Model file for the job. Use its own axes, mm. Round coordinates to 2 decimals unless told otherwise and drop trailing zeros. Loops run counter-clockwise (first coordinate to the right, second up) from the corner with the lowest first, then second, coordinate; pieces in that order, holes last. Notation, with made-up numbers: M 67.25,-37 L 87.25,-37 A20 cw 87.25,-8 Z; hole C -38,69.25 d10. An arc over 180 degrees is marked long. Use a Markdown table: item, result. Add a question column.
Item 1: Saw through at A-A on z = 2.6. Give the number of separate pieces and of enclosed holes in the cut face, then the cut area to 3 significant figures.
Item 2: Saw through at C-C on x = 109. Write the cut outline in (y, z).
Item 3: Pin check, flat tip, straight feed: P1, Ø2, axis at x = 92.5, z = 2, coming from the -Y side. Stop position of the tip, or through.
Item 4: Wall check: L1, parallel to X at y = -282.5, z = 1.5; L2, parallel to X at y = -127, z = 3.1 (3 decimals); L3, parallel to Y at x = 29.5, z = 0.7. Give the ranges that are in metal, low to high. Write a range as from..to.
Item 5: Saw through at B-B on x = 77. Write the cut outline in (y, z), then the cut area to 3 significant figures.
Autodesk Inventor part; units mm, degrees
ref_plane "YZ Plane" through (0, 0, 0) normal (1, 0, 0) x (0, 1, 0)
ref_plane "XZ Plane" through (0, 0, 0) normal (0, 1, 0) x (-1, 0, 0)
ref_plane "XY Plane" through (0, 0, 0) normal (0, 0, 1) x (1, 0, 0)
sketch "スケッチ1" plane through (0, 0, 0) normal (0, 0, 1) x (1, 0, 0)
  line L0 (0, 0) -> (150, 0)
  line L1 (150, 0) -> (150, -300)
  line L2 (150, -300) -> (0, -300)
  line L3 (0, -300) -> (0, 0)
  line L4 (150, -15) -> (0, -22.8612)
  circle A0 centre (130.1882, -77.2664) radius 1.75
  circle A1 centre (30.3252, -82.5) radius 1.75
  line L5 (130.1882, -77.2664) -> (30.3252, -82.5)
  dimension "d2" = 150
  dimension "d3" = 300
  dimension "d68" = 15
extrude "押し出し1" add sketch "スケッチ1" along normal blind 4 contours L4 L1 L2 L3 | A0 | A1
sketch "スケッチ2" plane through (0, 0, 0) normal (0, 0, -1) x (-1, 0, 0)
  line L0 (-125, -300) -> (-25, -300) construction
  line L1 (0, -300) -> (-150, -300)
  line L2 (-125, -307.5) -> (-25, -307.5)
  line L3 (-25, -292.5) -> (-125, -292.5)
  arc A0 (-125, -292.5) -> (-125, -307.5) centre (-125, -300) ccw
  arc A1 (-25, -307.5) -> (-25, -292.5) centre (-25, -300) ccw
  point P0 (0, 0)
  point P1 (-75, -300)
  point P2 (-132.5, -300)
  point P3 (-17.5, -300)
  dimension "d4" = 50
  dimension "d5" = 15
extrude "押し出し2" cut sketch "スケッチ2" against normal blind 4 contours L1 A0 L3 A1
fillet "フィレット1" radius 5 4 edges at (150, -300, 2) (132.5, -300, 2) (17.5, -300, 2) (0, -300, 2)
sketch "スケッチ3" plane through (0, 0, 0) normal (0, 0, -1) x (-1, 0, 0)
  line L0 (0, 0) -> (0, -295)
  line L1 (-125, -292.5) -> (-25, -292.5)
  line L2 (-129.863, -277.2664) -> (-30, -282.5)
  line L3 (-129.9354, -127.2664) -> (-30.0724, -132.5)
  line L4 (-129.884, -177.2664) -> (-30.021, -182.5)
  line L5 (-130.1882, -77.2664) -> (-30.3252, -82.5)
  line L6 (-150, 0) -> (0, 0)
  line L7 (-129.863, -227.2664) -> (-30, -232.5)
  dimension "d16" = 30
  dimension "d17" = 10
  dimension "d18" = 100
  dimension "d19" = 3
  dimension "d61" = 50
  dimension "d65" = 50
  dimension "d66" = 50
  dimension "d67" = 50
hole "穴1" at (30, -282.5, 0) at (129.863, -277.2664, 0) at (129.863, -227.2664, 0) at (129.9354, -127.2664, 0) at (30.0724, -132.5, 0) at (129.884, -177.2664, 0) at (30.021, -182.5, 0) at (130.1882, -77.2664, 0) at (30.3252, -82.5, 0) at (30, -232.5, 0) direction (0, 0, 1) diameter 3.5 end through all
fillet "フィレット2" radius 5 2 edges at (150, -15, 2) (0, -22.8612, 2)
properties part number "side_panel" material "木材(サクラ)"
Entries:
| question | item | result |
|---|---|---|
| 1 | separate pieces | 1 |
| 1 | enclosed holes | 10 |
| 1 | area | 41,200 mm2 |
| 2 | outline | M -292.5,0 L -17.15,0 L -17.15,4 L -292.5,4 Z |
| 3 | P1 | y = -292.5 |
| 4 | L1 | 0..28.25, 31.75..150 |
| 4 | L2 | 0..128.206, 131.665..150 |
| 4 | L3 | -292.5..-284.18, -280.82..-234.18, -230.82..-184.17, -180.83..-134.15, -130.85..-84.04, -80.96..-21.32 |
| 5 | outline | M -292.5,0 L -18.83,0 L -18.83,4 L -292.5,4 Z |
| 5 | area | 1,090 mm2 |
